Can you work these out from the model? Positions are in its coordinate system, mm. A direction names the side the tool comes from. Coordinates: 2 decimals unless noted, no trailing zeros. Order: outer loops, then holes, each group sorted by start corner. A loop starts at its lowest first (then second) coordinate and runs counter-clockwise, first axis right, second up. Notation, with made-up numbers: (72, 3.25) -> (106, 3.25) arc R30 cw to (106, 27.25) -> close; hole circle Ø1 at (-33, 63.5). An arc over 180 degrees is marked (long way). Return JSON: item names as keys, results as strings. Group by question number.
1) If we section it at A-A, the plane x = 0: Please give me the cut outline in (y, z), then the cut area to 3 significant figures.
2) For faces 4 (the flat face through (0, -76.2, 0)), 5 (the flat face through (0, 0, 13)), which set-ups out of +Z, -Z, +X, -X, +Y, -Y let a thin tool reach every point of the face, with its end or its side?
3) If we section it at B-B, the plane y = -34.5: Please give me the cut outline in (x, z), then the cut area to 3 significant figures.
4) For pin 1 (2 mm diameter, centred on x = 12, y = -24, fed in from +Z); pin 2 (7 mm diameter, centred on x = 0.5, z = 0, fed in from +Y); pin 3 (10 mm diameter, centred on x = 6, y = -29, fed in from -Z), each with a flat end and sliding along its axis, tell me the tip position at first contact or that it passes through.
5) Thinking about a two-plate mould opening in X: for faces 1 (the conical face through (-1.566, -7.672, -11.926)), 2 (the cylindrical face through (-9.55, -40.07, -12.46)), 3 (the flat face through (0, -81.28, 0)), which applies, +X half, -X half, draft (parallel to the pull), parting line (faces both ways), or undercut?
6) If we section it at C-C, the plane z = 0: Please give me the cut outline in (x, y), then the cut area to 3 significant figures.
7) If I drill on probe 1 along X at (y, z) = (-46.5, 0); probe 2 along X at (y, z) = (-73, -6); probe 3 along Y at (x, z) = (5, 7.5), over which ranges is the centre line in solid material (lowest first)? Write a range as from..to.
from build123d import *

# Parameters (mm, degrees)
SKETCH1_R           = 12.7
BOSS_EXTRUDE1_DEPTH = 12.7
BOSS_EXTRUDE1_DRAFT = -5
SKETCH2_R           = 3.175
CUT_EXTRUDE1_DEPTH  = 22.997045256
SKETCH7_R           = 1.27
CUT_EXTRUDE2_DEPTH  = 7.62
SKETCH10_R          = 15.7
BOSS_EXTRUDE2_DEPTH = 81.28
SKETCH11_R          = 12.7
CUT_EXTRUDE3_DEPTH  = 12.7
CUT_EXTRUDE3_DRAFT  = -5
SKETCH12_R          = 11.588893973
CUT_EXTRUDE4_DEPTH  = 63.5


with BuildPart() as part:
    # Sketch1 → Boss-Extrude1 (with draft: the straight prism first)
    with BuildSketch(Plane(origin=(0, 0, 0), x_dir=(1, 0, 0), z_dir=(0, 1, 0))):
        Circle(SKETCH1_R)
    extrude(amount=-BOSS_EXTRUDE1_DEPTH)
    # Boss-Extrude1: the draft: its side faces are tilted about the plane it starts from
    boss_extrude1_sides = [part.faces().sort_by_distance(p)[0] for p in [
        (-12.7, -6.35, 0),
    ]]
    draft(boss_extrude1_sides, Plane(origin=(0, 0, 0), x_dir=(1, 0, 0), z_dir=(0, 1, 0)), BOSS_EXTRUDE1_DRAFT)

    # Sketch2 → Cut-Extrude1 (cut, through all)
    with BuildSketch(Plane(origin=(0, 0, 0), x_dir=(1, 0, 0), z_dir=(0, 1, 0))):
        with Locations(Location((0, 0, 0), (0, 0, 270))):
            Circle(SKETCH2_R)
    extrude(amount=-CUT_EXTRUDE1_DEPTH, mode=Mode.SUBTRACT)

    # Sketch7 → Cut-Extrude2 (cut)
    with BuildSketch(Plane.XZ.offset(12.7)):
        with Locations(Location((-8.636, 0, 0), (0, 0, 270))):
            Circle(SKETCH7_R)
        with Locations(Location((4.318, 7.478995387, 0), (0, 0, 270))):
            Circle(SKETCH7_R)
    extrude(amount=-CUT_EXTRUDE2_DEPTH, mode=Mode.SUBTRACT)

    # Sketch10 → Boss-Extrude2 (add)
    with BuildSketch(Plane(origin=(0, 0, 0), x_dir=(1, 0, 0), z_dir=(0, 1, 0))):
        with Locations(Location((0, 0, 0), (0, 0, 270))):
            Circle(SKETCH10_R)
    extrude(amount=-BOSS_EXTRUDE2_DEPTH)


with BuildPart() as cut_extrude3_tool:
    # Sketch11 → Cut-Extrude3 (with draft: the straight prism first)
    with BuildSketch(Plane(origin=(0, 0, 0), x_dir=(1, 0, 0), z_dir=(0, 1, 0))):
        Circle(SKETCH11_R)
    extrude(amount=-CUT_EXTRUDE3_DEPTH)
    # Cut-Extrude3: the draft: its side faces are tilted about the plane it starts from
    cut_extrude3_sides = [cut_extrude3_tool.faces().sort_by_distance(p)[0] for p in [
        (-12.7, -6.35, 0),
    ]]
    draft(cut_extrude3_sides, Plane(origin=(0, 0, 0), x_dir=(1, 0, 0), z_dir=(0, 1, 0)), CUT_EXTRUDE3_DRAFT)


with BuildPart() as part_1:
    add(part.part)

    # Cut-Extrude3: cut by cut_extrude3_tool
    add(cut_extrude3_tool.part, mode=Mode.SUBTRACT)

    # Sketch12 → Cut-Extrude4 (cut)
    with BuildSketch(Plane(origin=(0, -12.7, 0), x_dir=(1, 0, 0), z_dir=(0, 1, 0))):
        with Locations(Location((0, 0, 0), (0, 0, 270))):
            Circle(SKETCH12_R)
    extrude(amount=-CUT_EXTRUDE4_DEPTH, mode=Mode.SUBTRACT)


solid = part_1.part
Result sheet:
{
 "1": {"outline": "(-81.28, -15.7) -> (0, -15.7) -> (0, -12.7) -> (-12.7, -11.59) -> (-76.2, -11.59) -> (-76.2, 11.59) -> (-12.7, 11.59) -> (0, 12.7) -> (0, 15.7) -> (-81.28, 15.7) -> close", "area": "772 mm2"},
 "2": {"face 4": "+Y", "face 5": "+Z, -Z, +X, -X, +Y"},
 "3": {"outline": "circle Ø31.4 at (0, 0); hole circle Ø23.18 at (0, 0)", "area": "352 mm2"},
 "4": {"pin 1": "stops at z = 11.2", "pin 2": "stops at y = -76.2", "pin 3": "stops at z = -15.67"},
 "5": {"face 1": "undercut", "face 2": "parting line", "face 3": "draft"},
 "6": {"outline": "(-15.7, -81.28) -> (15.7, -81.28) -> (15.7, 0) -> (12.7, 0) -> (11.59, -12.7) -> (11.59, -76.2) -> (-11.59, -76.2) -> (-11.59, -12.7) -> (-12.7, 0) -> (-15.7, 0) -> close", "area": "772 mm2"},
 "7": {"probe 1": "x = -15.7..-11.59, 11.59..15.7", "probe 2": "x = -14.51..-9.91, 9.91..14.51", "probe 3": "y = -81.28..-76.2"}
}
